```python
from build123d import *

# Parameters (mm, degrees)
BOSS_EXTRUDE1_DEPTH          = 6.35
F_10_0_1935_DIAMETER_HOLE1_D = 4.9149


with BuildPart() as part:
    # Sketch1 → Boss-Extrude1 (new body)
    with BuildSketch(Plane.XY):
        Polygon((0, 0), (-21.997045256, 12.7), (-21.997045256, 31.75), (0, 19.05), (50.8, 19.05), (50.8, 0), align=None)
    extrude(amount=BOSS_EXTRUDE1_DEPTH)

    # #10 (0.1935) Diameter Hole1 (through all)
    with Locations(Plane.XY.offset(6.35)):
        with Locations((44.45, 9.525), (25.4, 9.525)):
            Hole(F_10_0_1935_DIAMETER_HOLE1_D / 2)


solid = part.part
```
Check sheet for the modelled part. Datum: model origin and axes. Units: mm. Round coordinates to 2 decimals unless told otherwise and drop trailing zeros. Write each loop counter-clockwise with the first axis right and the second up, starting at its lowest first coordinate (ties: lowest second). Pieces come first, ordered by that corner, then holes. Notation, with made-up numbers: (65, -26.5) -> (119, -26.5) arc R19 ccw to (119, 4.5) -> close; hole circle Ø1 at (24.25, 16.5). An arc over 180 degrees is marked (long way). Put each result on its own line as item: value.
(1) Sectioned sample at B-B (y = 8.5). Enter the section's corners in (x, z).
Values found:
outline: (-14.72, 0) -> (23.17, 0) -> (23.17, 6.35) -> (-14.72, 6.35) -> close; (27.63, 0) -> (42.22, 0) -> (42.22, 6.35) -> (27.63, 6.35) -> close; (46.68, 0) -> (50.8, 0) -> (50.8, 6.35) -> (46.68, 6.35) -> close
(2) Sectioned sample at C-C (z = 4.25). Enter the section's corners in (x, y) (3 decimals).
Values found:
outline: (-21.997, 12.7) -> (0, 0) -> (50.8, 0) -> (50.8, 19.05) -> (0, 19.05) -> (-21.997, 31.75) -> close; hole circle Ø4.915 at (25.4, 9.525); hole circle Ø4.915 at (44.45, 9.525)
(3) Mould release check, pull along Y, two halves, no side actions. Record for faces 1 (the face through (27.855, 9.633, 3.131)), 2 (the face through (25, 19.05, 3)), 3 (the face through (15, 13, 6.35)): released by +Y, released by -Y, zero draft, split by the parting line, or undercut.
Values found:
face 1: undercut
face 2: released by +Y
face 3: zero draft
(4) Go/stop test with flat-tipped pins: pin 1 Ø8 at (x, y) = (44.45, 9.525) entering from +Z; pin 2 Ø4.5 at (x, y) = (25.4, 9.525) entering from +Z; pin 3 Ø3 at (x, z) = (23.5, 3.5) entering from +Y. Record where each tip stops, or that it passes through.
Values found:
pin 1: stops at z = 6.35
pin 2: passes through
pin 3: stops at y = 19.05
(5) Sectioned sample at A-A (x = 44.45). Enter the section's corners in (y, z), plus the area to 3 significant figures.
Values found:
outline: (0, 0) -> (7.07, 0) -> (7.07, 6.35) -> (0, 6.35) -> close; (11.98, 0) -> (19.05, 0) -> (19.05, 6.35) -> (11.98, 6.35) -> close
area: 89.8 mm^2
(6) Sectioned sample at D-D (x = 16). Enter the section's corners in (y, z).
Values found:
outline: (0, 0) -> (19.05, 0) -> (19.05, 6.35) -> (0, 6.35) -> close
(7) Material ranges on line 1 (Y direction, x = 25.4, z = 4); line 2 (X direction, y = 11.5, z = 0.75); line 3 (X direction, y = 10, z = 4.5), recorded low to high.
Values found:
line 1: y = 0 to 7.07, 11.98 to 19.05
line 2: x = -19.92 to 23.94, 26.86 to 42.99, 45.91 to 50.8
line 3: x = -17.32 to 22.99, 27.81 to 42.04, 46.86 to 50.8
